For this review, take the finished solid that the model builds, in its own axes (mm). Round coordinates to 2 decimals unless told otherwise and drop trailing zeros. Write each loop counter-clockwise with the first axis right and the second up, starting at its lowest first coordinate (ties: lowest second). Pieces come first, ordered by that corner, then holes. Notation, with made-up numbers: M 4,40 L 54,40 A14 ccw 54,61 Z; hole C 17.25,48.5 d3. An arc over 180 degrees is marked long. Use one line per item in the form item = value. Start each with the question number.
Item 1: Add section A-A (x = 0). State the section outline as (y, z) points, and give its area (3 significant figures).
Item 2: Add section C-C (x = -79). State the section outline as (y, z) points.
Item 3: Add section B-B (z = 79). State the section outline as (x, y) points, and give its area (3 significant figures).
Item 4: Add section D-D (z = 26.5). State the section outline as (x, y) points.
Item 5: For line 1 (X direction, y = 8.25, z = 0); line 2 (X direction, y = 6.75, z = 26); line 3 (X direction, y = 7.5, z = 26.5), list the stretches that pass through material, from the lowest coordinate up. Write a range as [from, to].
Item 6: For P1, Ø8.5, axis at x = -79, z = 0, coming from the -Y side; P2, Ø1, axis at y = 1, z = 26, coming from the +X side; P3, Ø5, axis at x = 9, y = 5.5, coming from the -Z side; P4, Ø1.5, axis at y = 6.5, z = 11, coming from the +X side, all flat-tipped, find the tip position at first contact; note any pin that passes through.
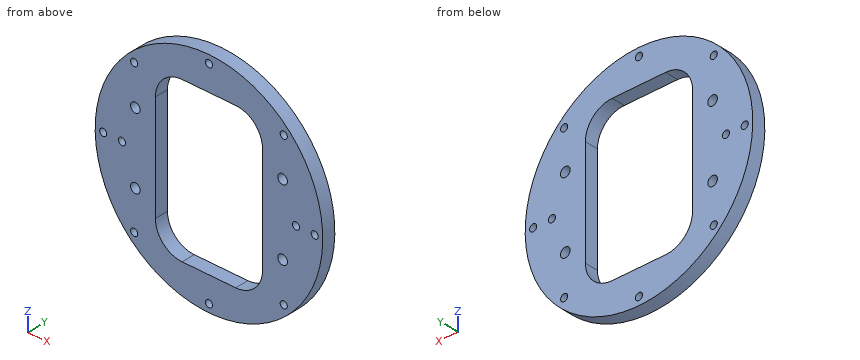
from build123d import *

# Parameters (mm, degrees)
SKETCH_1_R          = 85.5
SKETCH_1_R_2        = 2.65
SKETCH_1_W          = 80
SKETCH_1_H          = 100
EXTRUDE_3_DEPTH     = 10
SKETCH_10_R         = 3.6
SKETCH_10_R_2       = 2.65
CUT_EXTRUDE_2_DEPTH = 10
SKETCH_11_W         = 80
SKETCH_11_H         = 120
CUT_EXTRUDE_3_DEPTH = 10
FILLET_1_R          = 20
CUT_EXTRUDE_START   = -10
SKETCH_12_R         = 85.5
SKETCH_12_R_2       = 85
CUT_EXTRUDE_4_DEPTH = 10


with BuildPart() as part:
    # 草图1 → 凸台-拉伸3 (new body)
    with BuildSketch(Plane(origin=(0, 0, 0), x_dir=(1, 0, 0), z_dir=(0, 1, 0))):
        with Locations(Location((0, 0, 0), (0, 0, 270))):
            Circle(SKETCH_1_R)
        with Locations(Location((0, 79, 0), (0, 0, 270))):
            Circle(SKETCH_1_R_2, mode=Mode.SUBTRACT)
        with Locations(Location((55.861435714, 55.861435714, 0), (0, 0, 270))):
            Circle(SKETCH_1_R_2, mode=Mode.SUBTRACT)
        with Locations(Location((79, 0, 0), (0, 0, 270))):
            Circle(SKETCH_1_R_2, mode=Mode.SUBTRACT)
        with Locations(Location((55.861435714, -55.861435714, 0), (0, 0, 270))):
            Circle(SKETCH_1_R_2, mode=Mode.SUBTRACT)
        with Locations(Location((0, -79, 0), (0, 0, 270))):
            Circle(SKETCH_1_R_2, mode=Mode.SUBTRACT)
        with Locations(Location((-55.861435714, -55.861435714, 0), (0, 0, 270))):
            Circle(SKETCH_1_R_2, mode=Mode.SUBTRACT)
        with Locations(Location((-79, 0, 0), (0, 0, 270))):
            Circle(SKETCH_1_R_2, mode=Mode.SUBTRACT)
        with Locations(Location((-55.861435714, 55.861435714, 0), (0, 0, 270))):
            Circle(SKETCH_1_R_2, mode=Mode.SUBTRACT)
        Rectangle(SKETCH_1_W, SKETCH_1_H, mode=Mode.SUBTRACT)
    extrude(amount=EXTRUDE_3_DEPTH)

    # 草图10 → 切除-拉伸2 (cut)
    with BuildSketch(Plane(origin=(0, 10, 0), x_dir=(1, 0, 0), z_dir=(0, 1, 0))):
        with Locations(Location((55, 26.5, 0), (0, 0, 270))):
            Circle(SKETCH_10_R)
        with Locations(Location((65, 0, 0), (0, 0, 270))):
            Circle(SKETCH_10_R_2)
        with Locations(Location((55, -26.5, 0), (0, 0, 270))):
            Circle(SKETCH_10_R)
        with Locations(Location((-55, -26.5, 0), (0, 0, 270))):
            Circle(SKETCH_10_R)
        with Locations(Location((-55, 26.5, 0), (0, 0, 90))):
            Circle(SKETCH_10_R)
        with Locations(Location((-65, 0, 0), (0, 0, 270))):
            Circle(SKETCH_10_R_2)
    extrude(amount=-CUT_EXTRUDE_2_DEPTH, mode=Mode.SUBTRACT)

    # 草图11 → 切除-拉伸3 (cut)
    with BuildSketch(Plane(origin=(0, 10, 0), x_dir=(1, 0, 0), z_dir=(0, 1, 0))):
        Rectangle(SKETCH_11_W, SKETCH_11_H)
    extrude(amount=-CUT_EXTRUDE_3_DEPTH, mode=Mode.SUBTRACT)

    # 圆角1
    fillet_1_edges = [part.edges().sort_by_distance(p)[0] for p in [
        (40, 5, -60),
        (40, 5, 60),
        (-40, 5, 60),
        (-40, 5, -60),
    ]]
    fillet(fillet_1_edges, radius=FILLET_1_R)

    # 草图12 → 切除-拉伸4 (cut)
    with BuildSketch(Plane(origin=(0, 10, 0), x_dir=(1, 0, 0), z_dir=(0, 1, 0)).offset(CUT_EXTRUDE_START)):
        Circle(SKETCH_12_R)
        with Locations(Location((0, 0, 0), (0, 0, 270))):
            Circle(SKETCH_12_R_2, mode=Mode.SUBTRACT)
    extrude(amount=CUT_EXTRUDE_4_DEPTH, mode=Mode.SUBTRACT)


solid = part.part
Calculated:
q1.outline = M 0,-85 L 10,-85 L 10,-81.65 L 0,-81.65 Z; M 0,-76.35 L 10,-76.35 L 10,-60 L 0,-60 Z; M 0,60 L 10,60 L 10,76.35 L 0,76.35 Z; M 0,81.65 L 10,81.65 L 10,85 L 0,85 Z
q1.area = 394 mm^2
q2.outline = M 0,-31.37 L 10,-31.37 L 10,-2.65 L 0,-2.65 Z; M 0,2.65 L 10,2.65 L 10,31.37 L 0,31.37 Z
q3.outline = M -31.37,0 L -2.65,0 L -2.65,10 L -31.37,10 Z; M 2.65,0 L 31.37,0 L 31.37,10 L 2.65,10 Z
q3.area = 574 mm^2
q4.outline = M -80.76,0 L -58.6,0 L -58.6,10 L -80.76,10 Z; M -51.4,0 L -40,0 L -40,10 L -51.4,10 Z; M 40,0 L 51.4,0 L 51.4,10 L 40,10 Z; M 58.6,0 L 80.76,0 L 80.76,10 L 58.6,10 Z
q5.line_1 = [-85, -81.65], [-76.35, -67.65], [-62.35, -40], [40, 62.35], [67.65, 76.35], [81.65, 85]
q5.line_2 = [-80.93, -58.57], [-51.43, -40], [40, 51.43], [58.57, 80.93]
q5.line_3 = [-80.76, -58.6], [-51.4, -40], [40, 51.4], [58.6, 80.76]
q6.P1 = 0
q6.P2 = 81.08
q6.P3 = -84.75
q6.P4 = 84.38
